Verification items for the finished model (mm, model axes). A direction names the side the tool comes from. Give positions to 0.01 mm unless a question says otherwise; leave off trailing zeros. Write each loop counter-clockwise with the first axis right and the second up, starting at its lowest first coordinate (ties: lowest second). Pieces come first, ordered by that corner, then holes. Notation, with made-up numbers: (63.25, -35.75) -> (68.25, -35.75) arc R27 cw to (68.25, 0.25) -> close; hole circle Ø8 at (-0.5, -17). An arc over 180 degrees is marked (long way). Answer as CSV lines item,"result".
```python
from build123d import *

# Parameters (mm, degrees)
F0_W     = 240
F0_H     = 3
F1_DEPTH = 300
F3_DEPTH = 25
F4_W     = 240
F4_H     = 3
F5_DEPTH = 100
F6_R     = 3


with BuildPart() as f1:
    # F0 (on Front) → F1 (new body)
    with BuildSketch(Plane.XZ):
        Rectangle(F0_W, F0_H)
    extrude(amount=F1_DEPTH)

    # F2 (on face) → F3 (cut)
    with BuildSketch(Plane.XY.offset(1.5)):
        with BuildLine():
            ThreePointArc((-97.11, -25), (-99.61, -22.5), (-102.11, -25))
            Line((-102.11, -25), (-97.11, -25))
        make_face()
        with BuildLine():
            ThreePointArc((102.11, -25), (99.61, -22.5), (97.11, -25))
            Line((97.11, -25), (102.11, -25))
        make_face()
        with BuildLine():
            Line((102.11, -25), (97.11, -25))
            ThreePointArc((97.11, -25), (99.61, -27.5), (102.11, -25))
        make_face()
        with BuildLine():
            Line((-97.11, -25), (-102.11, -25))
            ThreePointArc((-102.11, -25), (-99.61, -27.5), (-97.11, -25))
        make_face()
        with BuildLine():
            ThreePointArc((-97.11, -235), (-99.61, -232.5), (-102.11, -235))
            Line((-102.11, -235), (-97.11, -235))
        make_face()
        with BuildLine():
            ThreePointArc((102.11, -235), (99.61, -232.5), (97.11, -235))
            Line((97.11, -235), (102.11, -235))
        make_face()
        with BuildLine():
            Line((102.11, -235), (97.11, -235))
            ThreePointArc((97.11, -235), (99.61, -237.5), (102.11, -235))
        make_face()
        with BuildLine():
            Line((-97.11, -235), (-102.11, -235))
            ThreePointArc((-102.11, -235), (-99.61, -237.5), (-97.11, -235))
        make_face()
    extrude(amount=-F3_DEPTH, mode=Mode.SUBTRACT)

    # F4 (on face) → F5 (join)
    with BuildSketch(Plane.XY.offset(1.5)):
        with Locations((0, -298.5)):
            Rectangle(F4_W, F4_H)
    extrude(amount=F5_DEPTH)

    # F6
    f6_edges = [f1.edges().sort_by_distance(p)[0] for p in [
        (0, -297, 1.5),
        (0, -300, -1.5),
    ]]
    fillet(f6_edges, radius=F6_R)


solid = f1.part
```
1) Section check A-A (x = -26). Record the boundary of the cut face in (y, z), and give its area (3 significant figures).
Reported:
outline,"(-300, 1.5) arc R3 ccw to (-297, -1.5) -> (0, -1.5) -> (0, 1.5) -> (-294, 1.5) arc R3 cw to (-297, 4.5) -> (-297, 101.5) -> (-300, 101.5) -> close"
area,"1,200 mm²"
2) Section check C-C (y = -206.5). Record the boundary of the cut face in (x, z), and give its area (3 significant figures).
Reported:
outline,"(-120, -1.5) -> (120, -1.5) -> (120, 1.5) -> (-120, 1.5) -> close"
area,"720 mm²"
3) Depth check by flat-ended pin: pin 1 (4 mm diameter, centred on x = 99.61, y = -25, fed in from +Z); pin 2 (3 mm diameter, centred on x = 76, y = -252, fed in from +Z); pin 3 (10 mm diameter, centred on x = 89.5, z = 37, fed in from +Y). Enter the tip coordinate at first touch or a pass-through.
Reported:
pin 1,"through"
pin 2,"z = 1.5"
pin 3,"y = -297"
4) Tool access check on faces 1 (the flat face through (-2, -297, 52)), 2 (the flat face through (-120, -151, 0)). Record the directions out of +Z, -Z, +X, -X, +Y, -Y that give a thin tool (end or side, any length) a straight path to the whole face; none if there is none.
Reported:
face 1,"+Z, +X, -X, +Y"
face 2,"+Z, -Z, -X, +Y, -Y"
5) Section check B-B (z = 75.5). Record the boundary of the cut face in (x, y).
Reported:
outline,"(-120, -300) -> (120, -300) -> (120, -297) -> (-120, -297) -> close"
6) Scan lines: line 1 along X through (y, z) = (-235, 0.5); line 2 along Y through (x, z) = (-99.61, 0.1); line 3 along Y through (x, z) = (99.61, 0.45). Record each from-to range of solid material in increasing order.
Reported:
line 1,"-120 to -102.11, -97.11 to 97.11, 102.11 to 120"
line 2,"-299.65 to -237.5, -232.5 to -27.5, -22.5 to 0"
line 3,"-299.81 to -237.5, -232.5 to -27.5, -22.5 to 0"
